Geometry check sheet. Reference: the model listing, model coordinates, mm. Face numbers are marked on the shaded views. A direction names the side the tool comes from. Give positions to 0.01 mm unless a question says otherwise; leave off trailing zeros. Loops run counter-clockwise (first coordinate to the right, second up) from the corner with the lowest first, then second, coordinate; pieces in that order, holes last. Notation, with made-up numbers: (-12, 66) -> (0, 66) arc R20 ccw to (0, 74) -> close; hole circle Ø11 at (10.25, -5.5). An arc over 180 degrees is marked (long way). Answer as a JSON object with one key per item and string values.
from build123d import *

# Parameters (mm, degrees)
SKETCH_2_W          = 16
SKETCH_2_H          = 40
EXTRUDE_1_DEPTH     = 2
EXTRUDE_START       = 1.5
SKETCH_4_R          = 2.6
EXTRUDE_2_DEPTH     = 3
FILLET_2_R          = 1.5
SKETCH_5_R          = 2.1
CUT_EXTRUDE_1_DEPTH = 34.763886032


with BuildPart() as part:
    # 草圖2 → 填料-伸長1 (new body)
    with BuildSketch(Plane(origin=(0, 0, 0), x_dir=(1, 0, 0), z_dir=(0, 1, 0))):
        Rectangle(SKETCH_2_W, SKETCH_2_H)
    extrude(amount=EXTRUDE_1_DEPTH)

    # 草圖4 → 填料-伸長2 (add)
    with BuildSketch(Plane.XY.offset(EXTRUDE_START)):
        with BuildLine():
            Line((8, 20), (8, 2))
            Line((8, 2), (-8, 2))
            Line((-8, 2), (-8, 20))
            ThreePointArc((-8, 20), (0, 28), (8, 20))
        make_face()
        with Locations((0, 20)):
            Circle(SKETCH_4_R, mode=Mode.SUBTRACT)
    extrude_2 = extrude(amount=EXTRUDE_2_DEPTH)

    # 鏡射1: 填料-伸長2 across plane
    add(extrude_2.mirror(Plane.XY))

    # 圓角2
    fillet_2_edges = [part.edges().sort_by_distance(p)[0] for p in [
        (0, 2, 4.5),
        (0, 2, 1.5),
        (0, 2, -4.5),
        (0, 2, -1.5),
    ]]
    fillet(fillet_2_edges, radius=FILLET_2_R - 0.0001)  # a hair under: the kernel refuses the full size

    # 草圖5 → 除料-伸長1 (cut, through all)
    with BuildSketch(Plane(origin=(0, 2, 0), x_dir=(1, 0, 0), z_dir=(0, 1, 0))):
        with Locations(Location((0, -12.5, 0), (0, 0, 270))):
            Circle(SKETCH_5_R)
        with Locations(Location((0, 12.5, 0), (0, 0, 90))):
            Circle(SKETCH_5_R)
    extrude(amount=-CUT_EXTRUDE_1_DEPTH, mode=Mode.SUBTRACT)


solid = part.part
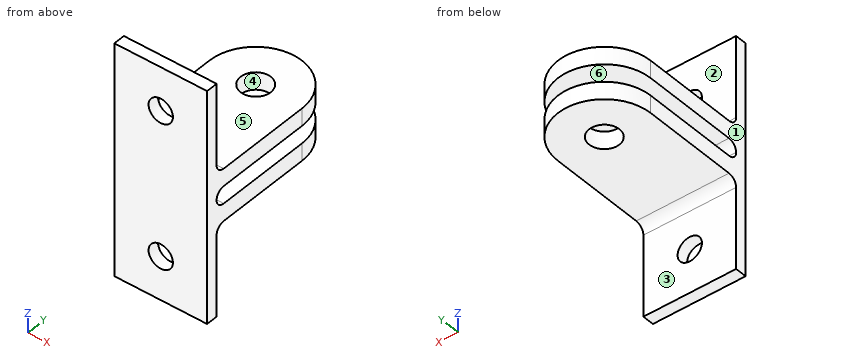
1) Section check C-C on y = 22. Record the cut outline in (x, z), plus the area to 3 significant figures.
Geometry check:
{"outline": "(-7.75, -4.5) -> (-1.66, -4.5) -> (-1.66, -1.5) -> (-7.75, -1.5) -> close; (-7.75, 1.5) -> (-1.66, 1.5) -> (-1.66, 4.5) -> (-7.75, 4.5) -> close; (1.66, -4.5) -> (7.75, -4.5) -> (7.75, -1.5) -> (1.66, -1.5) -> close; (1.66, 1.5) -> (7.75, 1.5) -> (7.75, 4.5) -> (1.66, 4.5) -> close", "area": "73.0 mm2"}
2) Section check A-A on z = 12.5. Record the cut outline in (x, y).
Geometry check:
{"outline": "(-8, 0) -> (-2.1, 0) -> (-2.1, 2) -> (-8, 2) -> close; (2.1, 0) -> (8, 0) -> (8, 2) -> (2.1, 2) -> close"}
3) Draft check along Z on the marked faces 4, 5 and 6. Enter one of: pulls with the +Z half, pulls with the -Z half, needs draft (parallel to the pull), parting line crosses it, or undercut.
Geometry check:
{"face 4": "needs draft", "face 5": "pulls with the +Z half", "face 6": "undercut"}
4) Tool access check on the marked faces 1, 2 and 3. Record the directions out of +Z, -Z, +X, -X, +Y, -Y that give a thin tool (end or side, any length) a straight path to the whole face; none if there is none.
Geometry check:
{"face 1": "+Z, -Z, -X, +Y, -Y", "face 2": "+Z, +X, -X, +Y", "face 3": "-Z, +X, -X, +Y"}
5) Depth check by flat-ended pin: P1, Ø8, axis at x = 3, y = 16, coming from the -Z side; P2, Ø5, axis at x = -3.5, y = 13.5, coming from the +Z side; P3, Ø7, axis at x = 0.5, z = -16, coming from the +Y side. Enter the tip coordinate at first touch or a pass-through.
Geometry check:
{"P1": "stops at z = -4.5", "P2": "stops at z = 4.5", "P3": "stops at y = 2"}
6) Material ranges on line 1 along Z through (x, y) = (-1.5, 6); line 2 along X through (y, z) = (1.4, -12.5); line 3 along Y through (x, z) = (7, 7.5), recorded low to high. Write a range as from..to.
Geometry check:
{"line 1": "z = -4.5..-1.5, 1.5..4.5", "line 2": "x = -8..-2.1, 2.1..8", "line 3": "y = 0..2"}
7) Section check B-B on y = 5.25. Record the cut outline in (x, z).
Geometry check:
{"outline": "(-8, -4.5) -> (8, -4.5) -> (8, -1.5) -> (-8, -1.5) -> close; (-8, 1.5) -> (8, 1.5) -> (8, 4.5) -> (-8, 4.5) -> close"}
